Can you work these out from the model? Positions are in its coordinate system, mm. Coordinates: 2 decimals unless noted, no trailing zeros. Write each loop counter-clockwise with the first axis right and the second up, starting at its lowest first coordinate (ties: lowest second). Pieces come first, ordered by that corner, then holes. Notation, with made-up numbers: M 21.25,-2 L 55.25,-2 A12 ccw 55.25,20 Z; hole C -40,-12 d9. An arc over 180 degrees is marked long. Use one line per item in the form item = value. Start each with the question number.
```python
from build123d import *

# Parameters (mm, degrees)
CHANFREIN1_SIZE   = 0.5
CHANFREIN1_SIZE_2 = 0.706151684


with BuildPart() as part:
    # Esquisse1 → Base-Révolution (revolve)
    with BuildSketch(Plane(origin=(0, 0, 0), x_dir=(1, 0, 0), z_dir=(0, 1, 0)), mode=Mode.PRIVATE) as base_r_volution_sk:
        with BuildLine():
            Line((0, 30), (0, 26.2))
            Line((0, 26.2), (4.422291236, 26.2))
            ThreePointArc((4.422291236, 26.2), (8, 27.8), (11.577708764, 26.2))
            Line((11.577708764, 26.2), (16, 26.2))
            Line((16, 26.2), (16, 30))
            ThreePointArc((16, 30), (15.707106781, 30.707106781), (15, 31))
            Line((15, 31), (1, 31))
            ThreePointArc((1, 31), (0.292893219, 30.707106781), (0, 30))
        make_face()
    revolve(base_r_volution_sk.sketch.rotate(Axis((0, 0, 0), (1, 0, 0)), 180), axis=Axis((0, 0, 0), (1, 0, 0)))

    # Esquisse2 → Enlèvement de matière-Révolution1 (revolve, cut)
    with BuildSketch(Plane.XY):
        with BuildLine():
            Line((0, 29.949958264), (0, 39.553831479))
            Line((0, 39.553831479), (16, 39.553831479))
            Line((16, 39.553831479), (16, 29.949958264))
            ThreePointArc((16, 29.949958264), (8, 31), (0, 29.949958264))
        make_face()
    revolve(axis=Axis((0, 0, 0), (1, 0, 0)), mode=Mode.SUBTRACT)

    # Chanfrein1
    # the kernel refuses this chamfer: 0.706151684, 0.5 mm, written as the material it takes off along each edge
    with BuildSketch(Plane(origin=(16, 0, 0), x_dir=(0, 1, 0), z_dir=(0, 0, -1))) as chanfrein1_piece_1:
        with BuildLine():
            Line((29.949958264 - CHANFREIN1_SIZE, 0), (30.121257319, -0.671299055))
            ThreePointArc((30.121257319, -0.671299055), (30.040483401, -0.34693806), (29.949958264, 0))
            Line((29.949958264, 0), (29.949958264 - CHANFREIN1_SIZE, 0))
        make_face()
    revolve(axis=Axis((16, 0, 0), (1, 0, 0)), mode=Mode.SUBTRACT)
    with BuildSketch(Plane(origin=(0, 0, 0), x_dir=(0, 1, 0), z_dir=(0, 0, -1))) as chanfrein1_piece_2:
        with BuildLine():
            Line((29.949958264 - CHANFREIN1_SIZE_2, 0), (30.074132004, 0.480253714))
            ThreePointArc((30.074132004, 0.480253714), (30.015483294, 0.249466944), (29.949958264, 0))
            Line((29.949958264, 0), (29.949958264 - CHANFREIN1_SIZE_2, 0))
        make_face()
    revolve(axis=Axis((0, 0, 0), (1, 0, 0)), mode=Mode.SUBTRACT)


solid = part.part
```
1) Will these pins go through, and if not, where does the flat tip stop? pin 1 Ø1.5 at (x, y) = (13, -16) entering from +Z; pin 2 Ø2 at (x, y) = (10.5, 23.5) entering from -Z; pin 3 Ø12 at (y, z) = (10, 13.5) entering from -X; pin 4 Ø1.5 at (x, y) = (4, 20) entering from -Z.
2) Suppose I cut it at C-C on x = 13.75. Please give me the cut outline in (y, z).
3) Suppose I cut it at D-D on x = 1.5. Please give me the cut outline in (y, z), and give its area (3 significant figures).
4) Please list where these lines run through material, in increasing order: line 1 (Z direction, x = 1, y = 7); line 2 (Z direction, x = 14, y = -15.5); line 3 (Y direction, x = 12.75, z = 8).
5) If we mould it in two halves opening along Z, with no side actions, what happens to faces 1 (the face through (2.24, -17.71, -19.31)), 2 (the face through (16, 2, 26.3)), 3 (the face through (13.82, -17.71, -19.31))? For each: +Z half, -Z half, draft (parallel to the pull), parting line (faces both ways), or undercut.
6) Suppose I cut it at A-A on z = 0. Please give me the cut outline in (x, y), and give its area (3 significant figures).
Computed values:
q1.pin_1 = 26.54
q1.pin_2 = -21.18
q1.pin_3 = through
q1.pin_4 = -23.98
q2.outline = C 0,0 d60.92; hole C 0,0 d52.4
q3.outline = C 0,0 d60.62; hole C 0,0 d52.4
q3.area = 730 mm²
q4.line_1 = -29.38 to -25.25, 25.25 to 29.38
q4.line_2 = -26.17 to -21.12, 21.12 to 26.17
q4.line_3 = -29.57 to -24.95, 24.95 to 29.57
q5.face_1 = undercut
q5.face_2 = draft
q5.face_3 = undercut
q6.outline = M 0,-29.24 L 0.48,-30.07 A31 ccw 15.33,-30.12 L 16,-29.45 L 16,-26.2 L 11.58,-26.2 A4.8 cw 4.42,-26.2 L 0,-26.2 Z; M 0,26.2 L 4.42,26.2 A4.8 cw 11.58,26.2 L 16,26.2 L 16,29.45 L 15.33,30.12 A31 ccw 0.48,30.07 L 0,29.24 Z
q6.area = 126 mm²
